Autodesk Fusion 360 part; units mm, degrees
sketch "Sketch1" plane through (0, 0, 0) normal (0, 0, 1) x (1, 0, 0)
  line L0 (0, 0) -> (64, 0)
  line L1 (64, 0) -> (64, 28)
  line L2 (64, 28) -> (0, 28)
  line L3 (0, 28) -> (0, 0)
  line L4 (0, 0) -> (0, 10)
  line L5 (0, 10) -> (64, 10)
  line L6 (32, 28) -> (42, 28)
  line L7 (32, 28) -> (22, 28)
  line L8 (22, 28) -> (42, 28)
  line L9 (42, 28) -> (42, 10)
  line L10 (42, 10) -> (22, 10)
  line L11 (22, 10) -> (22, 28)
  point P0 (32, 28)
  dimension "d1" = 64
  dimension "d2" = 28
  dimension "d3" = 10
extrude "Extrude1" add sketch "Sketch1" along normal blind 27.5
extrude "Extrude2" cut sketch "Sketch1" along normal blind 14.5 contours L0 L1 L3 L4 L5 L10
sketch "Sketch2" plane through (0, 0, 0) normal (0, -1, 0) x (1, 0, 0)
  line L0 (0, 14.5) -> (64, 14.5)
  line L1 (64, 14.5) -> (64, 27.5)
  line L2 (64, 27.5) -> (0, 27.5)
  line L3 (0, 27.5) -> (0, 14.5)
  line L4 (64, 14.5) -> (58, 14.5) construction
  line L5 (64, 14.5) -> (64, 20.5) construction
  line L6 (0, 14.5) -> (6, 14.5)
  line L7 (0, 14.5) -> (0, 20.5)
  point P0 (58, 20.5)
  point P1 (6, 20.5)
  dimension "d8" = 6
  dimension "d9" = 6
  dimension "d10" = 6
  dimension "d11" = 6
hole "Hole1" at (6, 0, 20.5) direction (0, 1, 0) diameter 3.4 depth 10 tip angle 118
hole "Hole2" at (58, 0, 20.5) direction (0, 1, 0) diameter 3.4 depth 10 tip angle 118
extrude "Extrude3" cut sketch "Sketch1" along normal blind 10 contours L2 L5 L6 L7 L8 L9 L10 L11
The listing builds one solid part. Answer for the finished solid, in the listing's coordinates (mm). A direction names the side the tool comes from. Coordinates: 2 decimals unless noted, no trailing zeros. Loops run counter-clockwise (first coordinate to the right, second up) from the corner with the lowest first, then second, coordinate; pieces in that order, holes last. Notation, with made-up numbers: (67, -28) - (104, -28) arc R20 cw to (104, -2) - close; hole circle Ø6 at (89.25, 1). An arc over 180 degrees is marked (long way). Use a Markdown table: item, result. Add a question column.
1) The mould has two halves that part along X. Classify faces 1 (the flat face through (11, 19, 0)), 2 (the flat face through (0, 17, 14)), 3 (the flat face through (42, 19, 5)), 4 (the flat face through (64, 17, 14)): released by +X, released by -X, zero draft, split by the parting line, or undercut.
2) Find the intervals of material crossed by line 1 (X direction, y = 3, z = 20.5); line 2 (Z direction, x = 58, y = 3); line 3 (X direction, y = 21.25, z = 7.5), in increasing order.
3) The part is cut by section C-C, the plane x = 52. Give the vertices of the cut face in (y, z), and give its area (3 significant figures).
4) The part is cut by section A-A, the plane z = 7.75. Give the vertices of the cut face in (x, y), and give its area (3 significant figures).
5) The part is cut by section B-B, the plane y = 22. Give the vertices of the cut face in (x, z).
6) Given pin 1 (3 mm diameter, centred on x = 24, y = 2.5, fed in from -Z); pin 2 (1.5 mm diameter, centred on x = 32.5, y = 11.5, fed in from -Z); pin 3 (2 mm diameter, centred on x = 58, z = 20.5, fed in from -Y), each flat-ended and moving along its own axis, determine where each tip first touches the part or whether it passes through.
7) For faces 5 (the flat face through (32, 14, 27.5)), 6 (the flat face through (32, 5, 14.5)), 7 (the flat face through (32, 28, 14)), 8 (the cylindrical face through (6.65, 5.07, 18.93)), 9 (the flat face through (32, 19, 10)), determine the directions among +Z, -Z, +X, -X, +Y, -Y from which every point of the face is accessible in a straight line to the end or side of a thin tool.
8) The part is cut by section D-D, the plane x = 34.5. Give the vertices of the cut face in (y, z), and give its area (3 significant figures).
Here are the results:
| question | item | result |
|---|---|---|
| 1 | face 1 | zero draft |
| 1 | face 2 | released by -X |
| 1 | face 3 | undercut |
| 1 | face 4 | released by +X |
| 2 | line 1 | x = 0 to 4.3, 7.7 to 56.3, 59.7 to 64 |
| 2 | line 2 | z = 14.5 to 18.8, 22.2 to 27.5 |
| 2 | line 3 | x = 0 to 22, 42 to 64 |
| 3 | outline | (0, 14.5) - (10, 14.5) - (10, 0) - (28, 0) - (28, 27.5) - (0, 27.5) - close |
| 3 | area | 625 mm^2 |
| 4 | outline | (0, 10) - (22, 10) - (22, 28) - (0, 28) - close; (42, 10) - (64, 10) - (64, 28) - (42, 28) - close |
| 4 | area | 792 mm^2 |
| 5 | outline | (0, 0) - (22, 0) - (22, 10) - (42, 10) - (42, 0) - (64, 0) - (64, 27.5) - (0, 27.5) - close |
| 6 | pin 1 | stops at z = 14.5 |
| 6 | pin 2 | stops at z = 10 |
| 6 | pin 3 | stops at y = 10.42 |
| 7 | face 5 | +Z, +X, -X, +Y, -Y |
| 7 | face 6 | -Z, +X, -X, -Y |
| 7 | face 7 | +Z, -Z, +X, -X, +Y |
| 7 | face 8 | -Y |
| 7 | face 9 | -Z, +Y, -Y |
| 8 | outline | (0, 14.5) - (10, 14.5) - (10, 10) - (28, 10) - (28, 27.5) - (0, 27.5) - close |
| 8 | area | 445 mm^2 |
